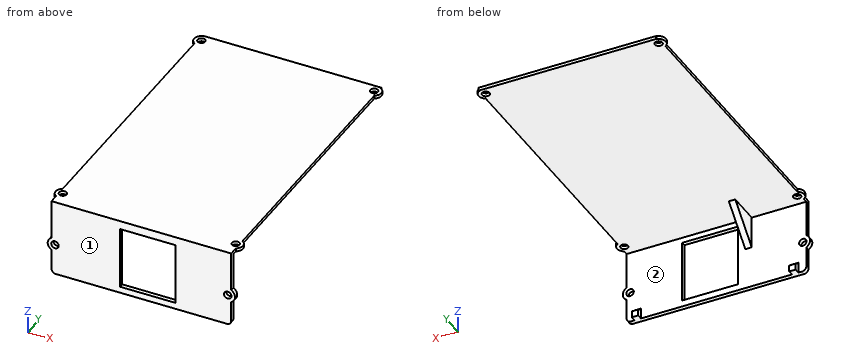
from build123d import *

# Parameters (mm, degrees)
SKETCH1_R                = 1.75
BOSS_EXTRUDE1_DEPTH      = 1.5
BOSS_EXTRUDE2_START      = -84
BOSS_EXTRUDE2_DEPTH      = 84
BOSS_EXTRUDE3_DEPTH      = 1.5
BOSS_EXTRUDE3_DEPTH_BACK = 1.5
BOSS_EXTRUDE4_DEPTH      = 2
SKETCH5_R                = 1.75
CUT_EXTRUDE1_DEPTH       = 2
CUT_EXTRUDE2_DEPTH       = 150.007183132
CUT_EXTRUDE2_DEPTH_BACK  = 150.007183132
SKETCH6_W                = 84
SKETCH6_H                = 5.379304891
BOSS_EXTRUDE6_START      = -2
SKETCH7_W                = 3
SKETCH7_H                = 4
BOSS_EXTRUDE6_DEPTH      = 2.5
FILLET1_R                = 2
CHAMFER1_SIZE            = 1
FILLET2_R                = 8
SKETCH8_W                = 26
SKETCH8_H                = 29.120695109
CUT_EXTRUDE3_DEPTH       = 22.4262221


with BuildPart() as part:
    # Sketch1 → Boss-Extrude1 (new body)
    with BuildSketch(Plane.XY):
        with BuildLine():
            Line((-38.75, -134.5), (38.75, -134.5))
            Line((38.75, -134.5), (42, -134.5))
            Line((42, -134.5), (42, -132.48653227))
            ThreePointArc((42, -132.48653227), (43.775, -129.5), (42, -126.51346773))
            Line((42, -126.51346773), (42, -6.48653227))
            ThreePointArc((42, -6.48653227), (43.741212037, -3.021861398), (41.104087703, -0.179091823))
            Line((41.104087703, -0.179091823), (42, 0))
            Line((42, 0), (-41, 0))
            Line((-41, 0), (-41.193033114, -0.199875483))
            ThreePointArc((-41.193033114, -0.199875483), (-43.747330957, -3.067121364), (-42, -6.48653227))
            Line((-42, -6.48653227), (-42, -126.51346773))
            ThreePointArc((-42, -126.51346773), (-43.775, -129.5), (-42, -132.48653227))
            Line((-42, -132.48653227), (-42, -134.5))
            Line((-42, -134.5), (-38.75, -134.5))
        make_face()
        with Locations((-40.375, -129.5)):
            Circle(SKETCH1_R, mode=Mode.SUBTRACT)
        with Locations((40.375, -129.5)):
            Circle(SKETCH1_R, mode=Mode.SUBTRACT)
        with Locations((40.375, -3.5)):
            Circle(SKETCH1_R, mode=Mode.SUBTRACT)
        with Locations((-40.375, -3.5)):
            Circle(SKETCH1_R, mode=Mode.SUBTRACT)
    extrude(amount=BOSS_EXTRUDE1_DEPTH)

    # Sketch2 → Boss-Extrude2 (add)
    with BuildSketch(Plane.ZY.offset(42).offset(BOSS_EXTRUDE2_START)):
        Polygon((1.5, -136.7), (1.5, -134.5), (0, -134.5), (0, -134.7), (-40, -134.7), (-40, -136.7), align=None)
    extrude(amount=BOSS_EXTRUDE2_DEPTH)

    # Sketch3 → Boss-Extrude3 (add, two sides: drawn at the far end of the back side and taken through both)
    with BuildSketch(Plane(origin=(-15, 0, 0), x_dir=(0, 0, -1), z_dir=(1, 0, 0)).offset(-BOSS_EXTRUDE3_DEPTH_BACK)):
        Polygon((0, -119.7), (15, -134.7), (0, -134.7), align=None)
    extrude(amount=BOSS_EXTRUDE3_DEPTH + BOSS_EXTRUDE3_DEPTH_BACK)

    # Sketch4 → Boss-Extrude4 (add)
    with BuildSketch(Plane.XZ.offset(136.7)):
        with BuildLine():
            Line((-42, -17.01346773), (-42, -22.98653227))
            ThreePointArc((-42, -22.98653227), (-43.775, -20), (-42, -17.01346773))
        make_face()
        with BuildLine():
            Line((42, -17.01346773), (42, -22.98653227))
            ThreePointArc((42, -22.98653227), (43.775, -20), (42, -17.01346773))
        make_face()
    extrude(amount=-BOSS_EXTRUDE4_DEPTH)

    # Sketch5 → Cut-Extrude1 (cut)
    with BuildSketch(Plane.XZ.offset(136.7)):
        with Locations(Location((40.375, -20, 0), (0, 0, 270))):
            Circle(SKETCH5_R)
        with Locations(Location((-40.375, -20, 0), (0, 0, 270))):
            Circle(SKETCH5_R)
    extrude(amount=-CUT_EXTRUDE1_DEPTH, mode=Mode.SUBTRACT)

    # Sketch6 → Cut-Extrude2 (cut, two sides: drawn at the far end of the back side and taken through both)
    with BuildSketch(Plane.XZ.offset(136.7).offset(-CUT_EXTRUDE2_DEPTH_BACK)):
        with Locations((0, -37.310347554)):
            Rectangle(SKETCH6_W, SKETCH6_H)
    extrude(amount=CUT_EXTRUDE2_DEPTH + CUT_EXTRUDE2_DEPTH_BACK, mode=Mode.SUBTRACT)

    # Sketch7 → Boss-Extrude6 (add)
    with BuildSketch(Plane.XZ.offset(136.7).offset(BOSS_EXTRUDE6_START)):
        with Locations((-36.8, -32.620695109)):
            Rectangle(SKETCH7_W, SKETCH7_H)
        with Locations((36.8, -32.620695109)):
            Rectangle(SKETCH7_W, SKETCH7_H)
    extrude(amount=-BOSS_EXTRUDE6_DEPTH)

    # Fillet1
    fillet1_edges = [part.edges().sort_by_distance(p)[0] for p in [
        (42, -135.7, -34.620695109),
        (-42, -135.7, -34.620695109),
    ]]
    fillet(fillet1_edges, radius=FILLET1_R)

    # Chamfer1
    chamfer1_edges = [part.edges().sort_by_distance(p)[0] for p in [
        (-36.8, -134.7, -30.620695109),
        (-36.8, -132.2, -30.620695109),
        (36.8, -134.7, -30.620695109),
        (36.8, -132.2, -30.620695109),
    ]]
    chamfer(chamfer1_edges, length=CHAMFER1_SIZE)

    # Fillet2
    # the kernel refuses this fillet: 8 mm, written as the material it takes off along each edge
    with BuildSketch(Plane(origin=(-30.303909917, -133.2, -30.620695109), x_dir=(0, -1.0, -1.111999381457983e-11), z_dir=(-1, 0, 0))) as fillet2_piece_1:
        with BuildLine():
            CenterArc((4.243746579, -7.06996192), FILLET2_R, 117.902496562, 17.097503438)
            Line((-1.413107671, -1.413107671), (0, 0))
            Line((0, 0), (0.5, 0))
        make_face()
    extrude(amount=12.992180166, mode=Mode.SUBTRACT)
    with BuildSketch(Plane(origin=(30.303909917, -133.2, -30.620695109), x_dir=(0, 0.7071067811865485, -0.7071067811865467), z_dir=(1, 0, 0))) as fillet2_piece_2:
        with BuildLine():
            CenterArc((1.998436033, -8), FILLET2_R, 90, 17.097503438)
            Line((-0.353553391, -0.353553391), (0, 0))
            Line((0, 0), (1.998436033, 0))
        make_face()
    extrude(amount=12.992180166, mode=Mode.SUBTRACT)

    # Sketch8 → Cut-Extrude3 (cut)
    with BuildSketch(Plane.XZ.offset(136.7)):
        with Locations((3, -17.060347555)):
            Rectangle(SKETCH8_W, SKETCH8_H)
    extrude(amount=-CUT_EXTRUDE3_DEPTH, mode=Mode.SUBTRACT)


solid = part.part
The model under review builds one solid part; all positions refer to its coordinate system, in mm. Face numbers are marked on the shaded views. A direction names the side the tool comes from. Round coordinates to 2 decimals unless told otherwise and drop trailing zeros. Loops run counter-clockwise (first coordinate to the right, second up) from the corner with the lowest first, then second, coordinate; pieces in that order, holes last. Notation, with made-up numbers: (86, 48) -> (93, 48) arc R28 ccw to (93, 70) -> close; hole circle Ø8 at (19, 56.5). An arc over 180 degrees is marked (long way). One line per question, with ' | ' between items. Start each with the question number.
Item 1: Wall thickness on line 1 along X through (y, z) = (-129.5, 0.9) (3 decimals); line 2 along Y through (x, z) = (34, -9); line 3 along Z through (x, y) = (-34.5, -114): over which ranges is each line inside the solid? List them lowest first. Write a range as [from, to].
Item 2: For pin 1 (0.8 mm diameter, centred on y = -133, z = -31.5, fed in from +X); pin 2 (1.6 mm diameter, centred on y = -135.5, z = -20.5, fed in from +X) (3 decimals); pin 3 (4.5 mm diameter, centred on x = 40.375, y = -129.5, fed in from -Z); pin 4 (4.5 mm diameter, centred on x = 40.375, z = -20, fed in from +Y), all flat-tipped, find the tip position at first contact; note any pin that passes through.
Item 3: Add section D-D, the plane x = -25. Write out the cut boundary in (y, z).
Item 4: Add section C-C, the plane y = -129.5. Write out the cut boundary in (x, z) (3 decimals).
Item 5: Add section B-B, the plane z = -13.5. Write out the cut boundary in (x, y), then the cut area to 4 significant figures.
Item 6: Machinability: for the marked faces 1 and 2, which of the approach directions +Z, -Z, +X, -X, +Y, -Y give a long, thin tool a straight path to every point of the face, cutting with its end or side? Answer none if there is none.
Item 7: Add section A-A, the plane z = -20. Write out the cut boundary in (x, y) (3 decimals), then the cut area to 3 significant figures.
Return value:
1) line 1: x = [-43.775, -42.125], [-38.625, 38.625], [42.125, 43.775] | line 2: y = [-136.7, -134.7] | line 3: z = [0, 1.5]
2) pin 1: stops at x = 38.3 | pin 2: stops at x = 43.775 | pin 3: stops at z = 0 | pin 4: stops at y = -134.7
3) outline: (-136.7, -34.62) -> (-134.7, -34.62) -> (-134.7, 0) -> (0, 0) -> (0, 1.5) -> (-136.7, 1.5) -> close
4) outline: (-43.775, 0) -> (-42.125, 0) -> (-42.125, 1.5) -> (-43.775, 1.5) -> close; (-38.625, 0) -> (-16.5, 0) -> (-16.5, -9.8) -> (-13.5, -9.8) -> (-13.5, 0) -> (38.625, 0) -> (38.625, 1.5) -> (-38.625, 1.5) -> close; (42.125, 0) -> (43.775, 0) -> (43.775, 1.5) -> (42.125, 1.5) -> close
5) outline: (-42, -136.7) -> (-10, -136.7) -> (-10, -134.7) -> (-13.5, -134.7) -> (-13.5, -133.2) -> (-16.5, -133.2) -> (-16.5, -134.7) -> (-42, -134.7) -> close; (16, -136.7) -> (42, -136.7) -> (42, -134.7) -> (16, -134.7) -> close | area: 120.5 mm2
6) face 1: +Z, -Z, +X, -X, -Y | face 2: +Y
7) outline: (-43.775, -136.7) -> (-42.125, -136.7) -> (-42.125, -134.7) -> (-43.775, -134.7) -> close; (-38.625, -136.7) -> (-10, -136.7) -> (-10, -134.7) -> (-38.625, -134.7) -> close; (16, -136.7) -> (38.625, -136.7) -> (38.625, -134.7) -> (16, -134.7) -> close; (42.125, -136.7) -> (43.775, -136.7) -> (43.775, -134.7) -> (42.125, -134.7) -> close | area: 109 mm2
